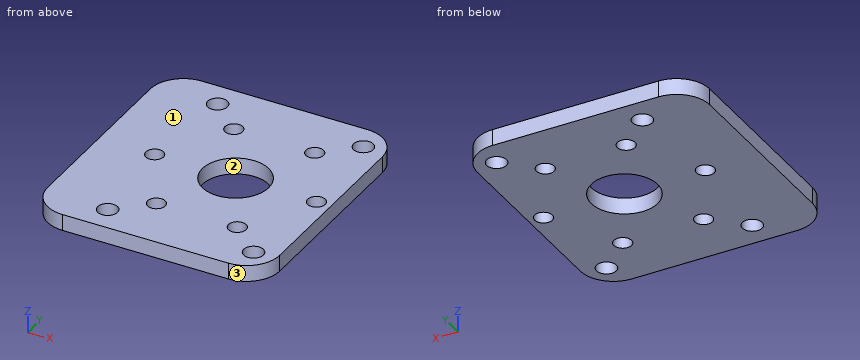
from build123d import *

# Parameters (mm, degrees)
SKETCH1_W                 = 44.45
SKETCH1_H                 = 48.26
BOSS_EXTRUDE1_DEPTH       = 3.1242
FILLET1_R                 = 6.35
F_6_CLEARANCE_HOLE1_D     = 3.7973
F_6_CLEARANCE_HOLE1_DEPTH = 5.08
F_6_CLEARANCE_HOLE1_TIP   = 1.140824014
SKETCH4_R                 = 6.35
CUT_EXTRUDE1_DEPTH        = 4.1242
M3_CLEARANCE_HOLE1_D      = 3.4


with BuildPart() as part:
    # Sketch1 → Boss-Extrude1 (new body)
    with BuildSketch(Plane.XY):
        with Locations((92.075, 24.13)):
            Rectangle(SKETCH1_W, SKETCH1_H)
    extrude(amount=BOSS_EXTRUDE1_DEPTH)

    # Fillet1
    fillet1_edges = [part.edges().sort_by_distance(p)[0] for p in [
        (69.85, 48.26, 1.5621),
        (114.3, 48.26, 1.5621),
        (114.3, 0, 1.5621),
        (69.85, 0, 1.5621),
    ]]
    fillet(fillet1_edges, radius=FILLET1_R)

    # #6 Clearance Hole1
    with Locations(Plane.XY.offset(3.1242)):
        with Locations((82.042, 43.18), (109.982, 43.18), (109.982, 5.08), (82.042, 5.08)):
            Hole(F_6_CLEARANCE_HOLE1_D / 2, depth=F_6_CLEARANCE_HOLE1_DEPTH)
            with Locations((0, 0, -(F_6_CLEARANCE_HOLE1_DEPTH + F_6_CLEARANCE_HOLE1_TIP / 2))):  # 118° drill point
                Cone(0, F_6_CLEARANCE_HOLE1_D / 2, F_6_CLEARANCE_HOLE1_TIP, mode=Mode.SUBTRACT)

    # Sketch4 → Cut-Extrude1 (cut, through all)
    with BuildSketch(Plane.XY.offset(3.1242)):
        with Locations((96.012, 24.13)):
            Circle(SKETCH4_R)
    extrude(amount=-CUT_EXTRUDE1_DEPTH, mode=Mode.SUBTRACT)

    # M3 Clearance Hole1 (through all)
    with Locations(Plane.XY.offset(3.1242)):
        with Locations((111.512, 24.13), (103.762, 10.706606241), (88.262, 10.706606241), (80.512, 24.13), (88.262, 37.553393759), (103.762, 37.553393759), (96.012, 24.13)):
            Hole(M3_CLEARANCE_HOLE1_D / 2)


solid = part.part
Design review of the part built by this model. Coordinates are the model's own, in mm. Face numbers are marked on the shaded views. Give positions to 0.01 mm unless a question says otherwise; leave off trailing zeros. Order: outer loops, then holes, each group sorted by start corner. A loop starts at its lowest first (then second) coordinate and runs counter-clockwise, first axis right, second up.
1. Add section A-A, the plane y = 24.13. State the section outline as (x, z) points, then the cut area to 3 significant figures.
Solution:
outline: (69.85, 0) - (78.81, 0) - (78.81, 3.12) - (69.85, 3.12) - close; (82.21, 0) - (89.66, 0) - (89.66, 3.12) - (82.21, 3.12) - close; (102.36, 0) - (109.81, 0) - (109.81, 3.12) - (102.36, 3.12) - close; (113.21, 0) - (114.3, 0) - (114.3, 3.12) - (113.21, 3.12) - close
area: 77.9 mm2
2. Add section B-B, the plane y = 4. State the section outline as (x, z) points.
Solution:
outline: (70.3, 0) - (80.48, 0) - (80.48, 3.12) - (70.3, 3.12) - close; (83.6, 0) - (108.42, 0) - (108.42, 3.12) - (83.6, 3.12) - close; (111.54, 0) - (113.85, 0) - (113.85, 3.12) - (111.54, 3.12) - close
3. Add section C-C, the plane x = 93.5. State the section outline as (y, z) points, then the cut area to 3 significant figures.
Solution:
outline: (0, 0) - (18.3, 0) - (18.3, 3.12) - (0, 3.12) - close; (29.96, 0) - (48.26, 0) - (48.26, 3.12) - (29.96, 3.12) - close
area: 114 mm2
4. Add section D-D, the plane x = 110.5. State the section outline as (y, z) points.
Solution:
outline: (0.53, 0) - (3.25, 0) - (3.25, 3.12) - (0.53, 3.12) - close; (6.91, 0) - (22.76, 0) - (22.76, 3.12) - (6.91, 3.12) - close; (25.5, 0) - (41.35, 0) - (41.35, 3.12) - (25.5, 3.12) - close; (45.01, 0) - (47.73, 0) - (47.73, 3.12) - (45.01, 3.12) - close
5. To check wall thickness, follow L1, parallel to Y at x = 89.5, z = 2.1; L2, parallel to Y at x = 80.5, z = 2.2; L3, parallel to Y at x = 81.5, z = 1.7. State the ranges of each line that lie inside material, in increasing order.
Solution:
L1: y = 0 to 9.54, 11.87 to 36.39, 38.72 to 48.26
L2: y = 0 to 3.97, 6.19 to 22.43, 25.83 to 42.07, 44.29 to 48.26
L3: y = 0 to 3.26, 6.9 to 22.75, 25.51 to 41.36, 45 to 48.26
6. Mouldability with a two-part tool opening along Y and no side actions: class the marked faces 1, 2 and 3 as +Y half, -Y half, draft (parallel to the pull), parting line (faces both ways), or undercut.
Solution:
face 1: draft
face 2: undercut
face 3: -Y half
